Part print with two shaded views. Sizes in mm from the minimum x, y, z corner. A direction names the side the tool comes from. Round coordinates to 2 decimals unless told otherwise and drop trailing zeros. Write each loop counter-clockwise with the first axis right and the second up, starting at its lowest first coordinate (ties: lowest second). Pieces come first, ordered by that corner, then holes. Notation, with made-up numbers: M 77,75.5 L 134,75.5 A21 ccw 134,88.5 Z; hole C 27.5,22 d1. An arc over 180 degrees is marked long. One line per question, with ' | ' between items. Start each with the question number.
1) Saw through at C-C (x = 8.5). List the corners of the cut face in (y, z).
2) Saw through at B-B (y = 1.5). Give the number of separate pieces and of enclosed holes in the cut face, plus the area to 3 significant figures.
3) Saw through at D-D (z = 38). List the corners of the cut face in (x, y), plus the area to 3 significant figures.
4) Saw through at A-A (z = 29.6). List the corners of the cut face in (x, y).
5) Wall check: probe 1 along X at (y, z) = (1.75, 30); probe 2 along Z at (x, y) = (57, 1); probe 3 along X at (y, z) = (3.25, 31.5). Give the ranges that are in metal, low to high. Write a range as [from, to].
6) Drop flat-ended pins along their axis: pin 1 Ø16.5 at (x, z) = (49, 10.2) entering from -Y; pin 2 Ø21 at (x, z) = (68.4, 10.2) entering from +Y; pin 3 Ø0.9 at (x, y) = (38, 7) entering from -Z; pin 4 Ø21 at (x, z) = (49, 29.6) entering from +Y. Give the stop position or say it passes through.
7) Tool access for the marked faces 1 and 2: list every direction of +Z, -Z, +X, -X, +Y, -Y with a clear straight run to the whole face (end or side of a thin tool).
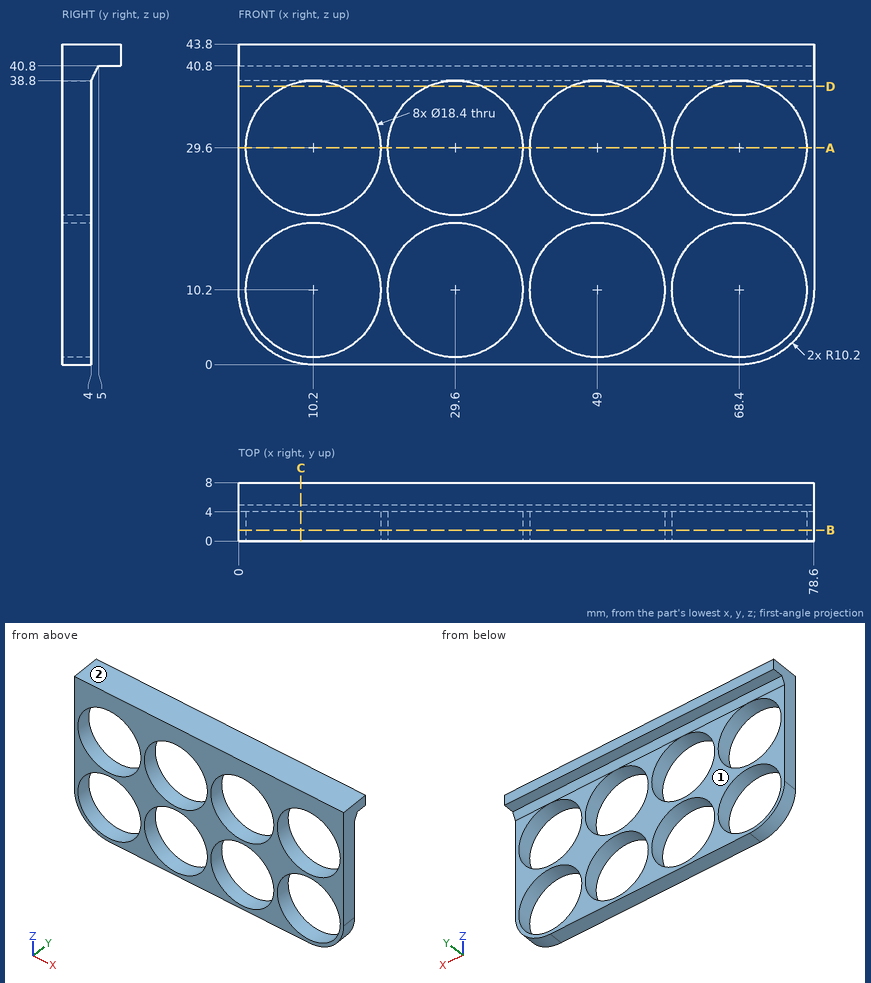
Answer key:
1) outline: M 0,0.14 L 4,0.14 L 4,1.16 L 0,1.16 Z; M 0,19.24 L 4,19.24 L 4,20.56 L 0,20.56 Z; M 0,38.64 L 4,38.64 L 4,38.8 L 5,40.8 L 8,40.8 L 8,43.8 L 0,43.8 Z
2) separate pieces: 1 | enclosed holes: 8 | area: 1,270 mm2
3) outline: M 0,0 L 6.45,0 L 6.45,4 L 0,4 Z; M 13.95,0 L 25.85,0 L 25.85,4 L 13.95,4 Z; M 33.35,0 L 45.25,0 L 45.25,4 L 33.35,4 Z; M 52.75,0 L 64.65,0 L 64.65,4 L 52.75,4 Z; M 72.15,0 L 78.6,0 L 78.6,4 L 72.15,4 Z | area: 194 mm2
4) outline: M 0,0 L 1,0 L 1,4 L 0,4 Z; M 19.4,0 L 20.4,0 L 20.4,4 L 19.4,4 Z; M 38.8,0 L 39.8,0 L 39.8,4 L 38.8,4 Z; M 58.2,0 L 59.2,0 L 59.2,4 L 58.2,4 Z; M 77.6,0 L 78.6,0 L 78.6,4 L 77.6,4 Z
5) probe 1: x = [0, 1.01], [19.39, 20.41], [38.79, 39.81], [58.19, 59.21], [77.59, 78.6] | probe 2: z = [0, 5.66], [14.74, 25.06], [34.14, 43.8] | probe 3: x = [0, 1.2], [19.2, 20.6], [38.6, 40], [58, 59.4], [77.4, 78.6]
6) pin 1: passes through | pin 2: stops at y = 4 | pin 3: stops at z = 40.8 | pin 4: stops at y = 4.65
7) face 1: -Z, +X, -X, +Y | face 2: +Z, +X, -X, +Y, -Y
